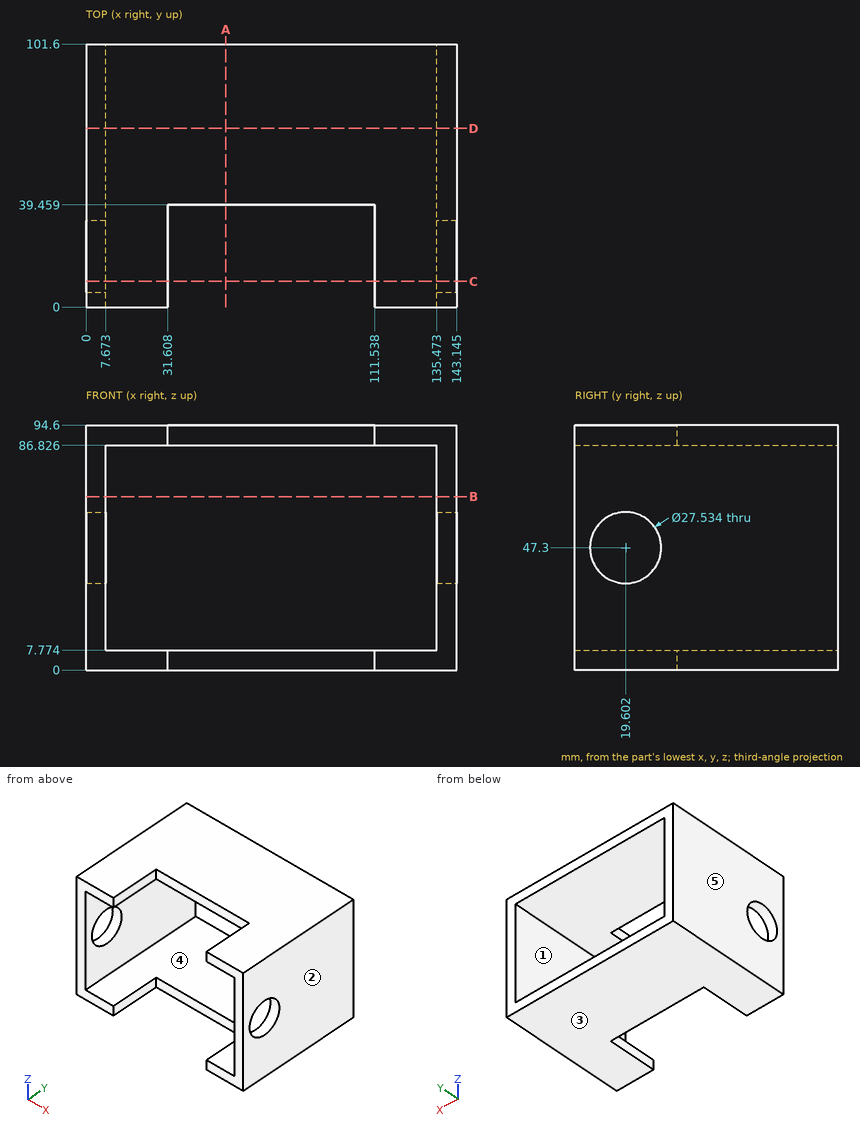
Design review of the part shown in the three views and the two pictorial views. Dimensions are in mm from the part's minimum x, y and z. A direction names the side the tool comes from. Coordinates: 2 decimals unless noted, no trailing zeros. Loops run counter-clockwise (first coordinate to the right, second up) from the corner with the lowest first, then second, coordinate; pieces in that order, holes last.
(1) Consider section A-A, the plane x = 54. Give the boundary of the cut face in (y, z) (1 decimal).
Determined:
outline: (39.5, 0) - (101.6, 0) - (101.6, 7.8) - (39.5, 7.8) - close; (39.5, 86.8) - (101.6, 86.8) - (101.6, 94.6) - (39.5, 94.6) - close
(2) Draft analysis for pull direction X (two halves, no side actions). For the marked faces 3, 4 and 5, state which applies: +X half, -X half, draft (parallel to the pull), parting line (faces both ways), or undercut.
Determined:
face 3: draft
face 4: undercut
face 5: -X half
(3) Consider section B-B, the plane z = 67. Give the boundary of the cut face in (x, y) (1 decimal), plus the area to 3 significant figures.
Determined:
outline: (0, 0) - (7.7, 0) - (7.7, 101.6) - (0, 101.6) - close; (135.5, 0) - (143.1, 0) - (143.1, 101.6) - (135.5, 101.6) - close
area: 1,560 mm2
(4) Consider section C-C, the plane y = 10. Give the boundary of the cut face in (x, z) (1 decimal).
Determined:
outline: (0, 0) - (31.6, 0) - (31.6, 7.8) - (7.7, 7.8) - (7.7, 37.4) - (0, 37.4) - close; (0, 57.2) - (7.7, 57.2) - (7.7, 86.8) - (31.6, 86.8) - (31.6, 94.6) - (0, 94.6) - close; (111.5, 0) - (143.1, 0) - (143.1, 37.4) - (135.5, 37.4) - (135.5, 7.8) - (111.5, 7.8) - close; (111.5, 86.8) - (135.5, 86.8) - (135.5, 57.2) - (143.1, 57.2) - (143.1, 94.6) - (111.5, 94.6) - close
(5) Insertion check: P1, Ø16.5, axis at y = 19.6, z = 47.3, coming from the +X side; P2, Ø8.5, axis at x = 76, z = 4.5, coming from the -Y side. Each pin has a flat end and moves straight along its axis. Give the tip position at first contact, or say it passes through.
Determined:
P1: passes through
P2: stops at y = 39.46
(6) Tool access review of the marked faces 1 and 2: name each direction out of +Z, -Z, +X, -X, +Y, -Y from which nothing blocks a thin tool from reaching the whole face with its end or side.
Determined:
face 1: +Y, -Y
face 2: +Z, -Z, +X, +Y, -Y
(7) Consider section D-D, the plane y = 69. Give the boundary of the cut face in (x, z) (1 decimal).
Determined:
outline: (0, 0) - (143.1, 0) - (143.1, 94.6) - (0, 94.6) - close; hole (7.7, 7.8) - (135.5, 7.8) - (135.5, 86.8) - (7.7, 86.8) - close
(8) Wall thickness on L1, parallel to Z at x = 112.5, y = 43 (1 decimal); L2, parallel to X at y = 27.5, z = 26.5 (1 decimal); L3, parallel to X at y = 31.5, z = 90 (1 decimal): over which ranges is each line inside the solid? List them lowest first.
Determined:
L1: z = 0 to 7.8, 86.8 to 94.6
L2: x = 0 to 7.7, 135.5 to 143.1
L3: x = 0 to 31.6, 111.5 to 143.1
